For this review, take the finished solid that the model builds, in its own axes (mm). Face numbers are marked on the shaded views. A direction names the side the tool comes from. Round coordinates to 2 decimals unless told otherwise and drop trailing zeros. Loops run counter-clockwise (first coordinate to the right, second up) from the corner with the lowest first, then second, coordinate; pieces in that order, holes last. Notation, with made-up numbers: M 86.25,37 L 130.25,37 A17 cw 130.25,48 Z; hole C 38.25,63.5 d6. An arc over 180 degrees is marked long. Write item = value, one per line. Start each with the question number.
```python
from build123d import *

# Parameters (mm, degrees)
F1_DEPTH = 76.2
F2_W     = 25.4
F2_H     = 74.0530890645
F3_DEPTH = 50.8


with BuildPart() as f1:
    # F0 (on Front) → F1 (new body)
    with BuildSketch(Plane.XZ):
        Polygon((-32.8333097622, 31.4650478065), (-32.8333097622, -32.0349521935), (30.6666902378, -32.0349521935), (-7.4333097622, 31.4650478065), align=None)
    extrude(amount=-F1_DEPTH)

    # F2 (on face) → F3 (join)
    with BuildSketch(Plane(origin=(8.4159697954, 0, 5.0495818772), x_dir=(0, 1, 0), z_dir=(0.8574929257, 0, 0.5144957554))):
        with Locations((38.1, -6.2210823096)):
            Rectangle(F2_W, F2_H)
    extrude(amount=F3_DEPTH)


solid = f1.part
```
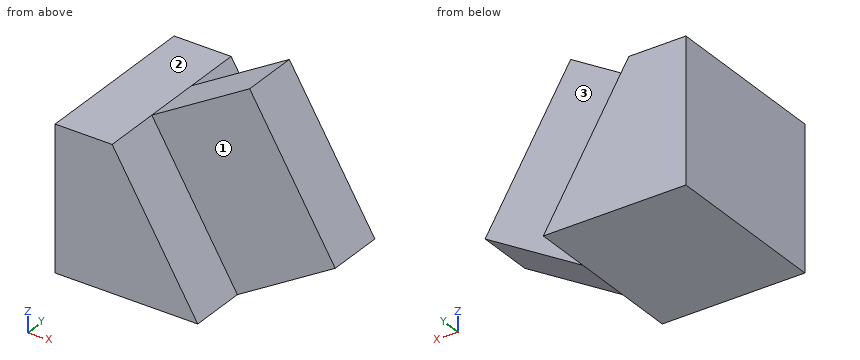
(1) For pin 1 Ø5 at (x, y) = (16.5, 10.5) entering from +Z; pin 2 Ø20.5 at (x, y) = (-14, 34.5) entering from +Z; pin 3 Ø3 at (x, z) = (63, 8.5) entering from -Y, all flat-tipped, find the tip position at first contact; note any pin that passes through.
(2) Tool access review of the marked faces 1, 2 and 3: name each direction out of +Z, -Z, +X, -X, +Y, -Y from which nothing blocks a thin tool from reaching the whole face with its end or side.
(3) Wall thickness on L1, parallel to Y at x = 26.5, z = -7; L2, parallel to Z at x = -8.5, y = 17; L3, parallel to Z at x = 39, y = 48.5: over which ranges is each line inside the solid? List them lowest first.
(4) Add section D-D on y = 9. Write out the cut boundary in (x, z).
(5) Add section C-C on y = 34. Write out the cut boundary in (x, z).
(6) Add section B-B on x = 25. Write out the cut boundary in (y, z).
(7) Add section A-A on z = 25. Write out the cut boundary in (x, y).
Answer sheet:
q1.pin_1 = -4.26
q1.pin_2 = 33.68
q1.pin_3 = 25.4
q2.face_1 = +Z, +X, -Y
q2.face_2 = +Z, -X, +Y, -Y
q2.face_3 = +Z, +X, +Y
q3.L1 = 25.4 to 50.8
q3.L2 = -32.03 to 31.47
q3.L3 = -27.03 to 52.81
q4.outline = M -32.83,-32.03 L 30.67,-32.03 L -7.43,31.47 L -32.83,31.47 Z
q5.outline = M -32.83,-32.03 L 30.67,-32.03 L 74.23,-5.9 L 36.13,57.6 L -7.43,31.47 L -32.83,31.47 Z
q6.outline = M 0,-32.03 L 76.2,-32.03 L 76.2,-22.59 L 50.8,-22.59 L 50.8,50.93 L 25.4,50.93 L 25.4,-22.59 L 0,-22.59 Z
q7.outline = M -32.83,0 L -3.55,0 L -3.55,25.4 L 55.69,25.4 L 55.69,50.8 L -3.55,50.8 L -3.55,76.2 L -32.83,76.2 Z
